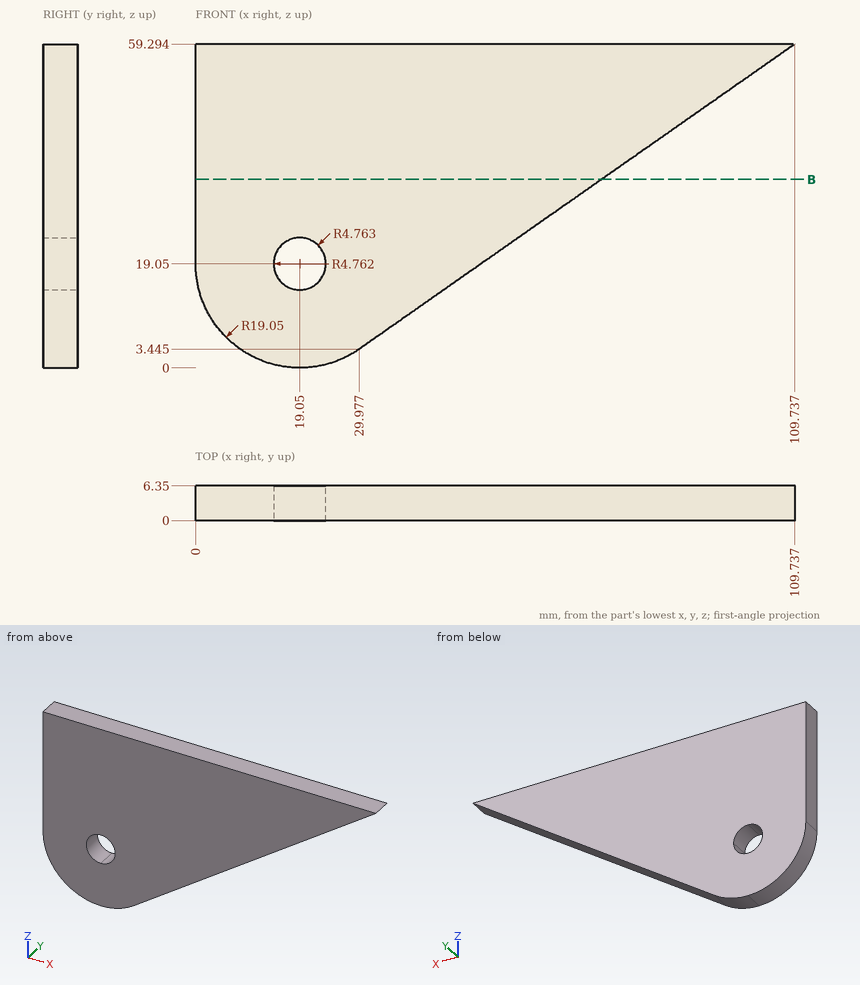
Source: three-view drawing plus pictorial views. Frame: mm from the lowest corner of the part. Coordinates: 2 decimals unless noted, no trailing zeros. Loops run counter-clockwise (first coordinate to the right, second up) from the corner with the lowest first, then second, coordinate; pieces in that order, holes last. Notation, with made-up numbers: (81.5, 70) - (120.5, 70) arc R8 ccw to (120.5, 74) - close; hole circle Ø1 at (67, 41). An arc over 180 degrees is marked (long way). Answer in a Markdown table with one row per item. Add a question column.
Item 1: Section query B-B on z = 34.5. Return the cut outline in (x, y), then the cut area to 3 significant figures.
Item 2: Contact query for flat-ended pins moving along their axis: P1, Ø1, axis at y = 1.5, z = 46, coming from the +X side (1 decimal); P2, Ø1, axis at x = 30, y = 3.5, coming from the -Z side. Output: stop coordinate, or through.
Item 3: Line query: line 1 along Z through (x, y) = (21, 0.5) (1 decimal); line 2 along Z through (x, y) = (20, 2.25) (1 decimal); line 3 along X through (y, z) = (2.5, 15.5) (1 decimal). Output: solid intervals per line, ascending. Write a range as [from, to].
Recorded:
| question | item | result |
|---|---|---|
| 1 | outline | (0, 0) - (74.33, 0) - (74.33, 6.35) - (0, 6.35) - close |
| 1 | area | 472 mm^2 |
| 2 | P1 | x = 91.5 |
| 2 | P2 | z = 3.12 |
| 3 | line 1 | [0.1, 14.7], [23.4, 59.3] |
| 3 | line 2 | [0, 14.4], [23.7, 59.3] |
| 3 | line 3 | [0.3, 15.9], [22.2, 47.2] |
